Could you check a few things on this drawing? It's one solid part, dimensions in mm from its lowest x, y, z. A direction names the side the tool comes from. Give positions to 0.01 mm unless a question says otherwise; leave off trailing zeros. Loops run counter-clockwise (first coordinate to the right, second up) from the corner with the lowest first, then second, coordinate; pieces in that order, holes last. Notation, with made-up numbers: M 41,52 L 88,52 A20 ccw 88,69 Z; hole C -9,17.25 d3. An arc over 180 degrees is marked long. Answer as a JSON object with one key per item and string values.
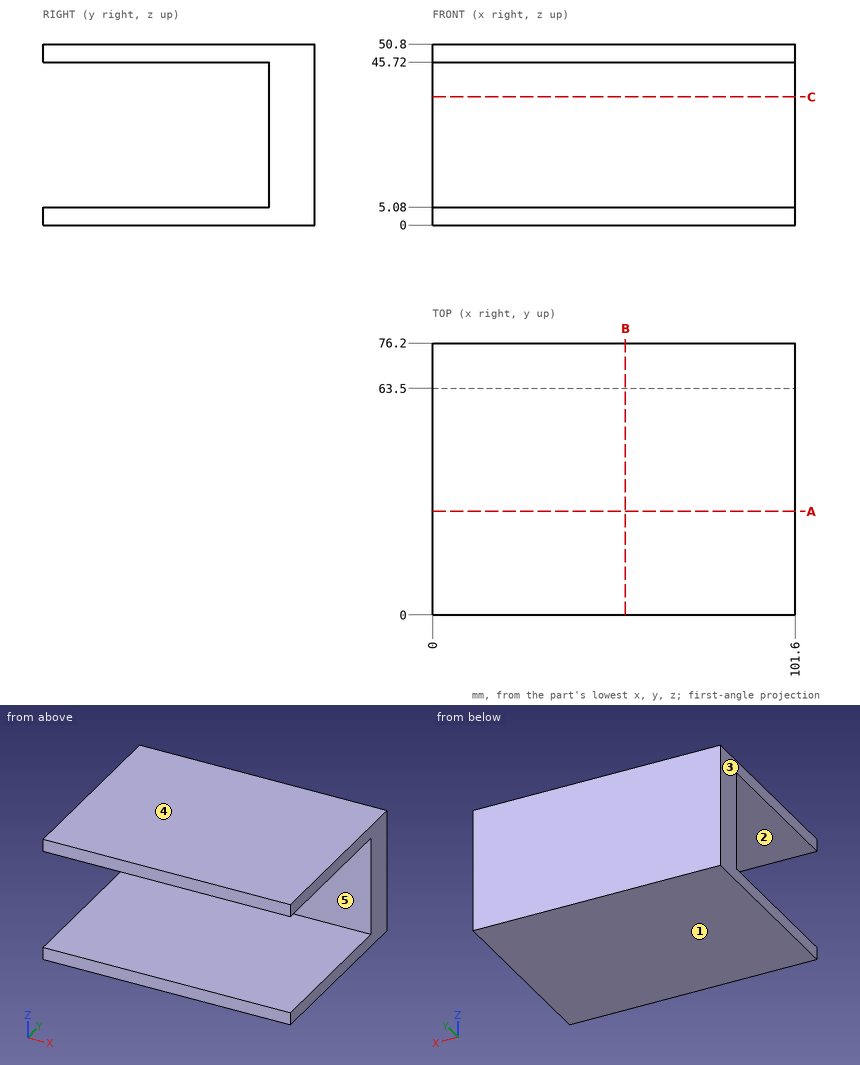
1) Suppose I cut it at C-C, the plane z = 36. Write out the boundary of the cut face in (x, y), and give its area (3 significant figures).
Answer list:
{"outline": "M 0,63.5 L 101.6,63.5 L 101.6,76.2 L 0,76.2 Z", "area": "1,290 mm^2"}
2) Suppose I cut it at A-A, the plane y = 29. Write out the boundary of the cut face in (x, z).
Answer list:
{"outline": "M 0,0 L 101.6,0 L 101.6,5.08 L 0,5.08 Z; M 0,45.72 L 101.6,45.72 L 101.6,50.8 L 0,50.8 Z"}
3) Will this pin go through, and if not, where does the flat tip stop? pin 1 Ø8 at (x, z) = (62, 19) entering from -Y.
Answer list:
{"pin 1": "y = 63.5"}
4) Please list where these lines run through material, in increasing order: line 1 along Z through (x, y) = (9.5, 7.5); line 2 along Y through (x, z) = (66, 26.5). Write a range as from..to.
Answer list:
{"line 1": "0..5.08, 45.72..50.8", "line 2": "63.5..76.2"}
5) For the marked faces 1 and 2, which set-ups out of +Z, -Z, +X, -X, +Y, -Y let a thin tool reach every point of the face, with its end or its side?
Answer list:
{"face 1": "-Z, +X, -X, +Y, -Y", "face 2": "+X, -X, -Y"}
6) Suppose I cut it at B-B, the plane x = 54. Write out the boundary of the cut face in (y, z), and give its area (3 significant figures).
Answer list:
{"outline": "M 0,0 L 76.2,0 L 76.2,50.8 L 0,50.8 L 0,45.72 L 63.5,45.72 L 63.5,5.08 L 0,5.08 Z", "area": "1,290 mm^2"}
7) If we mould it in two halves opening along Z, with no side actions, what happens to the marked faces 3, 4 and 5? For each: +Z half, -Z half, draft (parallel to the pull), parting line (faces both ways), or undercut.
Answer list:
{"face 3": "draft", "face 4": "+Z half", "face 5": "undercut"}
